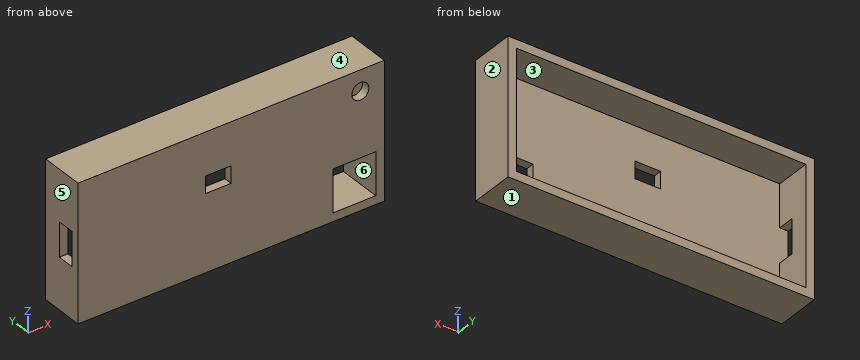
from build123d import *

# Parameters (mm, degrees)
SKETCH2_W           = 180
SKETCH2_H           = 80
SKETCH2_W_2         = 170
SKETCH2_H_2         = 70
BOSS_EXTRUDE1_DEPTH = 26
SKETCH2_4_W         = 70
SKETCH2_4_H         = 20
SKETCH2_4_W_2       = 15
SKETCH2_4_H_2       = 10
SKETCH2_4_R         = 5
BOSS_EXTRUDE2_DEPTH = 5
CUT_EXTRUDE1_DEPTH  = 5


with BuildPart() as part:
    # Sketch2 → Boss-Extrude1 (new body)
    with BuildSketch(Plane(origin=(0, 0, 0), x_dir=(1, 0, 0), z_dir=(0, 1, 0))):
        Rectangle(SKETCH2_W, SKETCH2_H)
        Rectangle(SKETCH2_W_2, SKETCH2_H_2, mode=Mode.SUBTRACT)
    extrude(amount=BOSS_EXTRUDE1_DEPTH)

    # Sketch2_4 → Boss-Extrude2 (add)
    # profile 1 of 2: a face of its own
    with BuildSketch(Plane(origin=(0, 0, 0), x_dir=(1, 0, 0), z_dir=(0, 1, 0))):
        with Locations((-50, -25)):
            Rectangle(SKETCH2_4_W, SKETCH2_4_H)
    # profile 2 of 2: a face of its own
    with BuildSketch(Plane(origin=(0, 0, 0), x_dir=(1, 0, 0), z_dir=(0, 1, 0))):
        Polygon((-15, -15), (-15, -35), (60, -35), (85, -35), (85, -10), (85, 10), (60, 10), (60, 35), (-85, 35), (-85, -15), align=None)
        with Locations((-7.5, -10)):
            Rectangle(SKETCH2_4_W_2, SKETCH2_4_H_2, mode=Mode.SUBTRACT)
        with Locations(Location((75.926069333, -27.828662368, 0), (0, 0, 270))):
            Circle(SKETCH2_4_R, mode=Mode.SUBTRACT)
    extrude(amount=BOSS_EXTRUDE2_DEPTH)

    # Sketch3 → Cut-Extrude1 (cut)
    with BuildSketch(Plane.ZY.offset(90)):
        Polygon((-10, 5), (0, 5), (0, 10), (0, 15), (-10, 15), align=None)
        Polygon((0, 10), (0, 5), (10, 5), (10, 15), (0, 15), align=None)
    extrude(amount=-CUT_EXTRUDE1_DEPTH, mode=Mode.SUBTRACT)


solid = part.part
Input: part model. Units: mm. Frame: model coordinates. Face numbers are marked on the shaded views. A direction names the side the tool comes from. Coordinates: 2 decimals unless noted, no trailing zeros. Loops run counter-clockwise (first coordinate to the right, second up) from the corner with the lowest first, then second, coordinate; pieces in that order, holes last.
(1) Section B-B on y = 17.75. Return the cut outline in (x, z).
(2) Section C-C on z = -4. Return the cut outline in (x, y).
(3) Pull-direction query (Z, two-part tool) for the marked faces 1, 2, 3 and 4; classes: released by +Z, released by -Z, zero draft, split by the parting line, or undercut.
(4) Material intervals for probe 1 along X at (y, z) = (6, -24.5); probe 2 along Z at (x, y) = (-57, 17); probe 3 along X at (y, z) = (4.25, -15), sorted ascending.
(5) First-contact query: pin 1 Ø1 at (x, z) = (46.5, 25.5) entering from +Y. Flat tip, straight axial feed; report the tip coordinate or a pass-through.
(6) Set-up query: the marked faces 5 and 6. Return all of +Z, -Z, +X, -X, +Y, -Y with unobstructed straight access to the full face (end or side cutting, diameter ignored); none if empty.
(7) Section A-A on z = 12. Return the cut outline in (x, y).
(8) Section D-D on x = -63. Return the cut outline in (y, z), then the cut area to 3 significant figures.
Data:
1. outline: (-90, -40) - (90, -40) - (90, 40) - (-90, 40) - close; hole (-85, -35) - (85, -35) - (85, 35) - (-85, 35) - close
2. outline: (-90, 0) - (90, 0) - (90, 26) - (85, 26) - (85, 5) - (-90, 5) - close; (-90, 15) - (-85, 15) - (-85, 26) - (-90, 26) - close
3. face 1: released by -Z
3. face 2: zero draft
3. face 3: undercut
3. face 4: released by +Z
4. probe 1: x = -90 to -85, 85 to 90
4. probe 2: z = -40 to -35, 35 to 40
4. probe 3: x = -90 to 60, 85 to 90
5. pin 1: stops at y = 5
6. face 5: +Z, -Z, -X, +Y, -Y
6. face 6: +Y
7. outline: (-90, 0) - (-15, 0) - (-15, 5) - (-85, 5) - (-85, 26) - (-90, 26) - close; (0, 0) - (90, 0) - (90, 26) - (85, 26) - (85, 5) - (0, 5) - close
8. outline: (0, -40) - (26, -40) - (26, -35) - (5, -35) - (5, 35) - (26, 35) - (26, 40) - (0, 40) - close
8. area: 610 mm2
